Answer from the drawing. Dimensions are ordinates in mm from the lowest x, y and z of the part. A direction names the side the tool comes from. Round coordinates to 2 decimals unless told otherwise and drop trailing zeros. Order: outer loops, then holes, each group sorted by start corner. A loop starts at its lowest first (then second) coordinate and runs counter-clockwise, first axis right, second up.
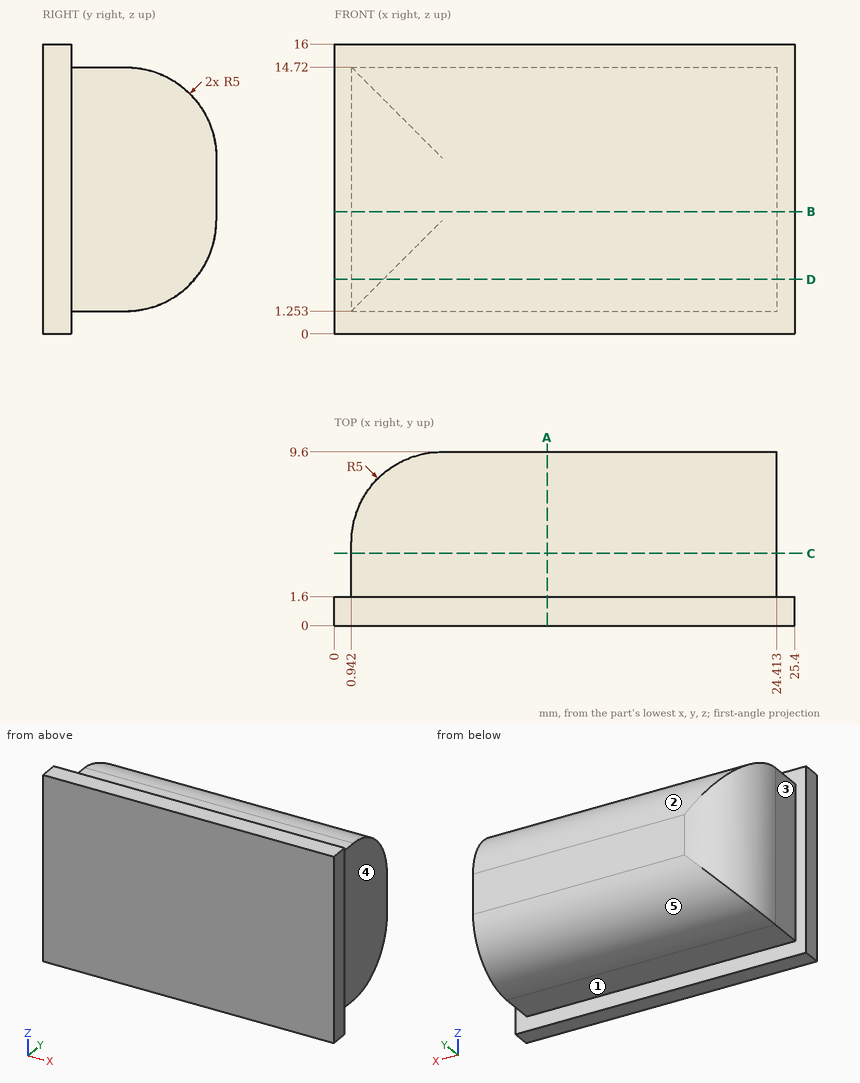
Q1. For the marked faces 4 and 5, determine the directions among +Z, -Z, +X, -X, +Y, -Y from which every point of the face is accessible in a straight line to the end or side of a thin tool.
Outcome:
face 4: +Z, -Z, +X, +Y
face 5: -Z, +X, -X, +Y
Q2. Straight lines are drawn through the part: probe 1 along Y at (x, z) = (10, 6); probe 2 along Z at (x, y) = (23.25, 3); probe 3 along X at (y, z) = (2.5, 4.25). For each, find the intervals that lie inside material, in ascending order.
Outcome:
probe 1: y = 0 to 9.59
probe 2: z = 1.25 to 14.72
probe 3: x = 0.94 to 24.41
Q3. Flat-ended cylindrical pins translate along their axes: pin 1 (0.9 mm diameter, centred on x = 8, y = 3.5, fed in from -Z); pin 2 (4 mm diameter, centred on x = 20, z = 4, fed in from -Y); pin 3 (0.9 mm diameter, centred on x = 16, y = 3, fed in from +Z); pin 4 (4 mm diameter, centred on y = 6, z = 4.5, fed in from +X). Find the tip coordinate at first contact, or state that the pin passes through.
Outcome:
pin 1: stops at z = 1.25
pin 2: stops at y = 0
pin 3: stops at z = 14.72
pin 4: stops at x = 24.41
Q4. A cutting plane is placed at C-C, the plane y = 4. Give the vertices of the cut face in (x, z), plus the area to 3 significant figures.
Outcome:
outline: (0.94, 1.25) - (24.41, 1.25) - (24.41, 14.72) - (0.94, 14.72) - close
area: 316 mm2
Q5. For a pull along Z with two mould halves and no side action, classify the marked faces 1, 2 and 3 as released by +Z, released by -Z, zero draft, split by the parting line, or undercut.
Outcome:
face 1: released by -Z
face 2: released by +Z
face 3: zero draft
Q6. A cutting plane is placed at B-B, the plane z = 6.75. Give the vertices of the cut face in (x, y), plus the area to 3 significant figures.
Outcome:
outline: (0, 0) - (25.4, 0) - (25.4, 1.6) - (24.41, 1.6) - (24.41, 9.6) - (5.94, 9.6) arc R5 ccw to (0.94, 4.6) - (0.94, 1.6) - (0, 1.6) - close
area: 223 mm2
Q7. A cutting plane is placed at D-D, the plane z = 3. Give the vertices of the cut face in (x, y).
Outcome:
outline: (0, 0) - (25.4, 0) - (25.4, 1.6) - (24.41, 1.6) - (24.41, 8.4) - (2.69, 8.4) arc R5 ccw to (0.94, 4.6) - (0.94, 1.6) - (0, 1.6) - close
Q8. A cutting plane is placed at A-A, the plane x = 11.75. Give the vertices of the cut face in (y, z).
Outcome:
outline: (0, 0) - (1.6, 0) - (1.6, 1.25) - (4.6, 1.25) arc R5 ccw to (9.6, 6.25) - (9.6, 9.72) arc R5 ccw to (4.6, 14.72) - (1.6, 14.72) - (1.6, 16) - (0, 16) - close
